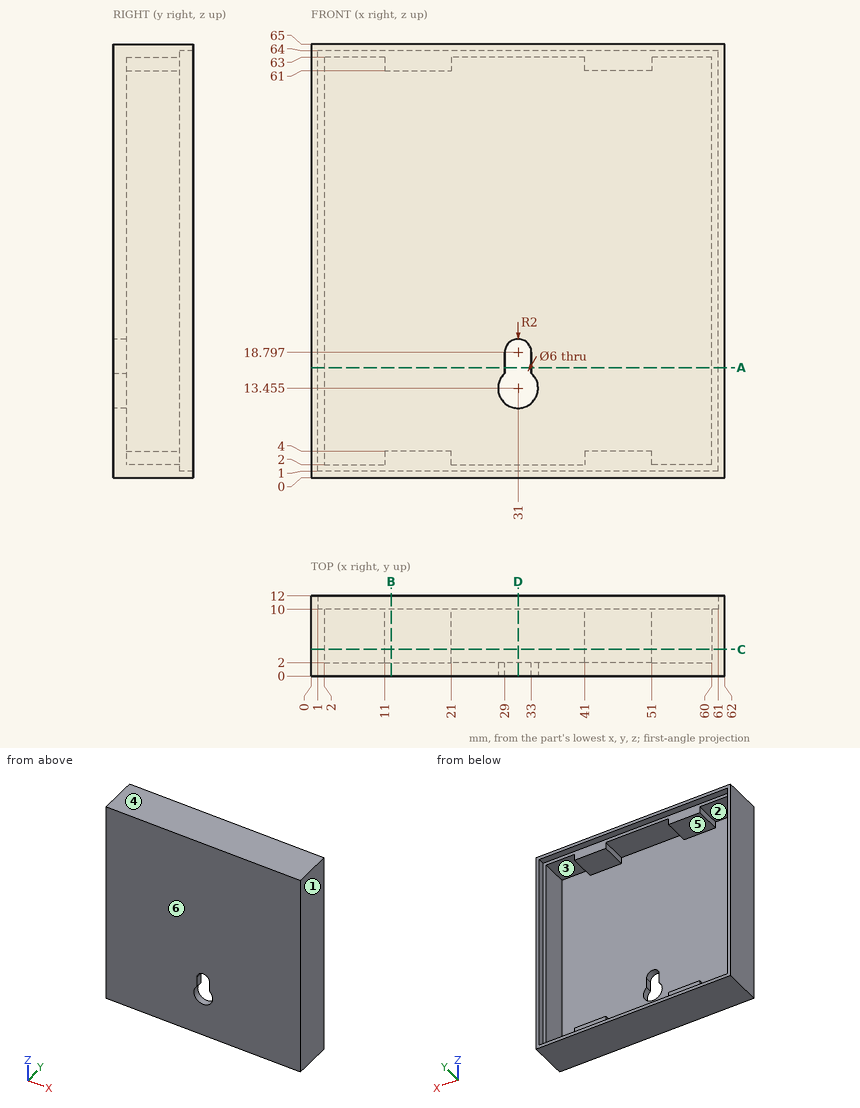
Print and shaded views of the part. All mm, measured from the part's lowest x, y and z. A direction names the side the tool comes from. Coordinates: 2 decimals unless noted, no trailing zeros. Order: outer loops, then holes, each group sorted by start corner. A loop starts at its lowest first (then second) coordinate and runs counter-clockwise, first axis right, second up. Notation, with made-up numbers: M 1.25,17 L 9.25,17 A24 cw 9.25,42 Z; hole C 29,-38.75 d11. An arc over 180 degrees is marked long. Answer as CSV lines item,"result".
1) Drill centre lines: L1, parallel to X at y = 9.25, z = 62; L2, parallel to X at y = 5, z = 25; L3, parallel to Z at x = 36, y = 2.25. Where is each one in solid material? Low to high. Write a range as from..to.
Verdict:
L1,"0..2, 11..21, 41..51, 60..62"
L2,"0..2, 60..62"
L3,"0..2, 63..65"
2) Mould opens along Z. For the marked faces 1, 2, 3 and 4 say: released by +Z, released by -Z, zero draft, split by the parting line, or undercut.
Verdict:
face 1,"zero draft"
face 2,"undercut"
face 3,"undercut"
face 4,"released by +Z"
3) Cut at D-D (x = 31). List the corners of the cut face in (y, z) (1 decimal), then the cut area to 3 significant figures.
Verdict:
outline,"M 0,0 L 12,0 L 12,1 L 10,1 L 10,2 L 2,2 L 2,10.5 L 0,10.5 Z; M 0,20.8 L 2,20.8 L 2,63 L 10,63 L 10,64 L 12,64 L 12,65 L 0,65 Z"
area,"145 mm2"
4) Cut at C-C (y = 4). List the corners of the cut face in (x, z), then the cut area to 3 significant figures.
Verdict:
outline,"M 0,0 L 62,0 L 62,65 L 0,65 Z; hole M 2,2 L 11,2 L 11,4 L 21,4 L 21,2 L 41,2 L 41,4 L 51,4 L 51,2 L 60,2 L 60,63 L 51,63 L 51,61 L 41,61 L 41,63 L 21,63 L 21,61 L 11,61 L 11,63 L 2,63 Z"
area,"572 mm2"
5) Cut at B-B (x = 12). List the corners of the cut face in (y, z), then the cut area to 3 significant figures.
Verdict:
outline,"M 0,0 L 12,0 L 12,1 L 10,1 L 10,4 L 2,4 L 2,61 L 10,61 L 10,64 L 12,64 L 12,65 L 0,65 Z"
area,"198 mm2"
6) 3-axis set-ups, long thin cutter, end or side, ignore diameter. For the marked faces 5 and 6: which of +Z, -Z, +X, -X, +Y, -Y reach the whole face in a straight line?
Verdict:
face 5,"+Y"
face 6,"+Z, -Z, +X, -X, -Y"
7) Cut at A-A (z = 16.5). List the corners of the cut face in (x, y), then the cut area to 3 significant figures.
Verdict:
outline,"M 0,0 L 29,0 L 29,2 L 2,2 L 2,10 L 1,10 L 1,12 L 0,12 Z; M 33,0 L 62,0 L 62,12 L 61,12 L 61,10 L 60,10 L 60,2 L 33,2 Z"
area,"152 mm2"
8) Flat gauge pin, fed straight in: P1, Ø18, axis at x = 45, z = 38.5, coming from the +Y side. Where does the tip first touch, or does it go through?
Verdict:
P1,"y = 2"
